Build history of the part. All positions in model axes, mm. A direction names the side the tool comes from. Round coordinates to 2 decimals unless told otherwise and drop trailing zeros. Write each loop counter-clockwise with the first axis right and the second up, starting at its lowest first coordinate (ties: lowest second). Pieces come first, ordered by that corner, then holes. Notation, with made-up numbers: M 33,26.25 L 88,26.25 A24 ccw 88,63.25 Z; hole C 80,53.25 d6. An arc over 180 degrees is marked long. Write item = value, one per line.
from build123d import *

# Parameters (mm, degrees)
PAD_DEPTH   = 100
SKETCH002_R = 45
HOLE_DEPTH  = 12


with BuildPart() as part:
    # Sketch → Revolution (revolve)
    with BuildSketch(Plane.XZ):
        with BuildLine():
            ThreePointArc((10, 0), (24.813455, 49.126357), (31.5, 100))
            Line((31.5, 100), (24.5, 100))
            Line((24.5, 100), (24.5, 95))
            Line((24.5, 95), (26.5, 95))
            ThreePointArc((0, 26), (18.469352, 58.495466), (26.5, 95))
            Line((0, 26), (0, 0))
            Line((0, 0), (10, 0))
        make_face()
    revolve(axis=Axis((0, 0, 0), (0, 0, 1)))

    # Sketch001 (on Face1 of Revolution) → Pad (new body)
    with BuildSketch(Plane(origin=(0, 0, 0), x_dir=(1, 0, 0), z_dir=(0, 0, -1))):
        Polygon((-3, 18), (-21, 0), (-21, -6), (-9, -18), (9, -18), (21, -6), (21, 0), (3, 18), align=None)
    extrude(amount=PAD_DEPTH)

    # Sketch002 (on Face9 of Pad) → Hole (cut)
    with BuildSketch(Plane(origin=(0, 18, 0), x_dir=(1, 0, 0), z_dir=(0, 1, 0))):
        with Locations((0, 50)):
            Circle(SKETCH002_R)
    extrude(amount=-HOLE_DEPTH, mode=Mode.SUBTRACT)


with BuildPart() as part_1:
    # Body placement: moved
    add(part.part.moved(Location((0, 0, -26))))


solid = part_1.part
1. Band-saw the part on B-B (y = 13). Count the separate pieces of the cut face and the enclosed holes in it, plus the area to 3 significant figures.
Responses:
separate_pieces = 3
enclosed_holes = 0
area = 2,250 mm²
2. Flat gauge pins, fed straight in: pin 1 (1 mm diameter, centred on y = -6.5, z = -57.5, fed in from +X); pin 2 (1 mm diameter, centred on y = -4, z = -35, fed in from -X); pin 3 (2 mm diameter, centred on x = 15.5, z = -76.5, fed in from -Y). Where does each tip first touch, or does it go through?
Responses:
pin_1 = 15
pin_2 = -17.5
pin_3 = -6.5
3. Tool access for faces 1 (the face through (0, 11, -121)), 2 (the face through (-15, 12, -122)), 3 (the face through (0, 12, -26)), 4 (the face through (21, 3, -75)): list every direction of +Z, -Z, +X, -X, +Y, -Y with a clear straight run to the whole face (end or side of a thin tool).
Responses:
face_1 = +Y
face_2 = -Z, -X, +Y
face_3 = none
face_4 = -Z, +X, +Y, -Y
4. Band-saw the part on A-A (z = -48). List the corners of the cut face in (x, y), plus the area to 3 significant figures.
Responses:
outline = M -21,0 L -3,-18 L 3,-18 L 21,0 L 21,6 L -21,6 Z
area = 684 mm²
5. Mould opens along Z. For faces 5 (the face through (0, 4, -126)), 6 (the face through (0, 11, -31)), 7 (the face through (16, -19, 74)), 8 (the face through (0, 18, -123)) say: pulls with the +Z half, pulls with the -Z half, needs draft (parallel to the pull), parting line crosses it, or undercut.
Responses:
face_5 = pulls with the -Z half
face_6 = undercut
face_7 = pulls with the +Z half
face_8 = needs draft
6. Probe probe 1 along Y at (x, z) = (-8, 38); probe 2 along Y at (x, z) = (0, 72.75); probe 3 along X at (y, z) = (-12, -116). List the from-to ranges inside material, lowest first.
Responses:
probe_1 = -26.46 to -18.81, 18.81 to 26.46
probe_2 = -31.44 to -24.5, 24.5 to 31.44
probe_3 = -9 to 9
